from build123d import *

# Parameters (mm, degrees)
SKETCH1_W           = 120
SKETCH1_H           = 120
SKETCH1_W_2         = 80
SKETCH1_H_2         = 80
BOSS_EXTRUDE1_DEPTH = 20
SKETCH2_W           = 20
SKETCH2_H           = 20
BOSS_EXTRUDE2_DEPTH = 450
SKETCH4_W           = 120
SKETCH4_H           = 120
SKETCH4_W_2         = 80
SKETCH4_H_2         = 80
BOSS_EXTRUDE3_DEPTH = 20


with BuildPart() as part:
    # Sketch1 → Boss-Extrude1 (new body)
    with BuildSketch(Plane(origin=(0, 0, 0), x_dir=(1, 0, 0), z_dir=(0, 1, 0))):
        Rectangle(SKETCH1_W, SKETCH1_H)
        Rectangle(SKETCH1_W_2, SKETCH1_H_2, mode=Mode.SUBTRACT)
    extrude(amount=BOSS_EXTRUDE1_DEPTH)

    # Sketch2 → Boss-Extrude2 (add)
    with BuildSketch(Plane(origin=(0, 450, 0), x_dir=(1, 0, 0), z_dir=(0, 1, 0))):
        with Locations((-50, 50)):
            Rectangle(SKETCH2_W, SKETCH2_H)
        with Locations((50, 50)):
            Rectangle(SKETCH2_W, SKETCH2_H)
        with Locations((50, -50)):
            Rectangle(SKETCH2_W, SKETCH2_H)
        with Locations((-50, -50)):
            Rectangle(SKETCH2_W, SKETCH2_H)
    extrude(amount=-BOSS_EXTRUDE2_DEPTH)

    # Sketch4 → Boss-Extrude3 (add)
    with BuildSketch(Plane(origin=(0, 450, 0), x_dir=(1, 0, 0), z_dir=(0, 1, 0))):
        Rectangle(SKETCH4_W, SKETCH4_H)
        Rectangle(SKETCH4_W_2, SKETCH4_H_2, mode=Mode.SUBTRACT)
    extrude(amount=-BOSS_EXTRUDE3_DEPTH)


solid = part.part
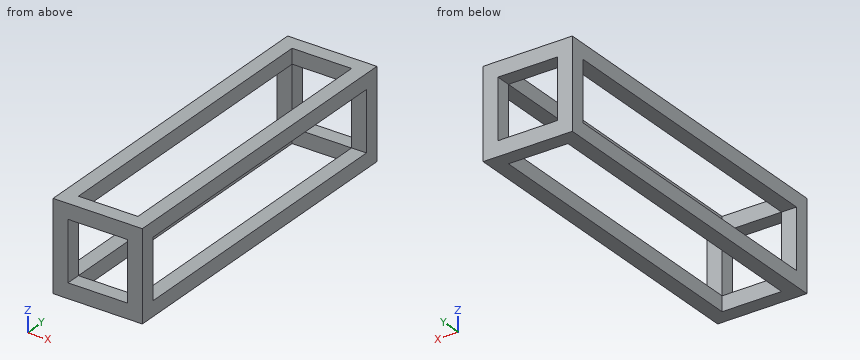
Work out the finished part from the listing and answer in its coordinate system (mm). Give positions to 0.01 mm unless a question says otherwise; leave off trailing zeros. Order: outer loops, then holes, each group sorted by start corner. A loop starts at its lowest first (then second) coordinate and runs counter-clockwise, first axis right, second up. Notation, with made-up numbers: M 73,26 L 106,26 A22 cw 106,37 Z; hole C 84,7.5 d10. An arc over 180 degrees is marked long. Return JSON: item names as keys, results as strings.
Q1. Find section A-A, the plane z = -25. Write down the section's boundary in (x, y).
Answer below:
{"outline": "M -60,0 L -40,0 L -40,20 L -60,20 Z; M -60,430 L -40,430 L -40,450 L -60,450 Z; M 40,0 L 60,0 L 60,20 L 40,20 Z; M 40,430 L 60,430 L 60,450 L 40,450 Z"}
Q2. Find section D-D, the plane z = -46.5. Write down the section's boundary in (x, y).
Answer below:
{"outline": "M -60,0 L 60,0 L 60,450 L -60,450 Z; hole M -40,20 L 40,20 L 40,430 L -40,430 Z"}
Q3. Find section C-C, the plane y = 361.5. Write down the section's boundary in (x, z), and give its area (3 significant figures).
Answer below:
{"outline": "M -60,-60 L -40,-60 L -40,-40 L -60,-40 Z; M -60,40 L -40,40 L -40,60 L -60,60 Z; M 40,-60 L 60,-60 L 60,-40 L 40,-40 Z; M 40,40 L 60,40 L 60,60 L 40,60 Z", "area": "1,600 mm^2"}
Q4. Find the intervals of material crossed by line 1 along Y through (x, z) = (2, 42); line 2 along X through (y, z) = (124.5, -50), in increasing order. Write a range as [from, to].
Answer below:
{"line 1": "y = [0, 20], [430, 450]", "line 2": "x = [-60, -40], [40, 60]"}
Q5. Find section B-B, the plane x = 50. Write down the section's boundary in (y, z), and give its area (3 significant figures).
Answer below:
{"outline": "M 0,-60 L 450,-60 L 450,60 L 0,60 Z; hole M 20,-40 L 430,-40 L 430,40 L 20,40 Z", "area": "21,200 mm^2"}
